Input: part model. Units: mm. Frame: model coordinates. Face numbers are marked on the shaded views. A direction names the side the tool comes from. Coordinates: 2 decimals unless noted, no trailing zeros. Order: outer loops, then holes, each group sorted by start corner. A loop starts at its lowest first (then second) coordinate and runs counter-clockwise, first axis right, second up. Notation, with made-up numbers: (15.25, 6) -> (48.25, 6) arc R8 cw to (48.25, 17) -> close; hole circle Ø8 at (85, 64). An arc over 180 degrees is marked (long way). One line per item, written item: value. Start each with the question number.
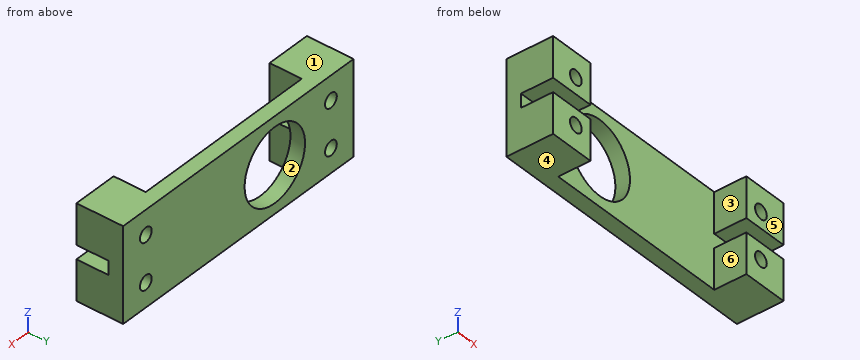
from build123d import *

# Parameters (mm, degrees)
SKETCH2_W           = 61
SKETCH2_H           = 20.5
SKETCH2_R           = 8
SKETCH2_R_2         = 1.55
BOSS_EXTRUDE1_DEPTH = 3.175
SKETCH3_W           = 9.85
SKETCH3_H           = 8.75
SKETCH3_R           = 1.55
BOSS_EXTRUDE2_DEPTH = 7


with BuildPart() as part:
    # Sketch2 → Boss-Extrude1 (new body)
    with BuildSketch(Plane(origin=(0, 0, 0), x_dir=(1, 0, 0), z_dir=(0, 1, 0))):
        Rectangle(SKETCH2_W, SKETCH2_H)
        with Locations((-9.65, 0)):
            Circle(SKETCH2_R, mode=Mode.SUBTRACT)
        with Locations((-24.5, 5)):
            Circle(SKETCH2_R_2, mode=Mode.SUBTRACT)
        with Locations((-24.5, -5)):
            Circle(SKETCH2_R_2, mode=Mode.SUBTRACT)
        with Locations((24.5, 5)):
            Circle(SKETCH2_R_2, mode=Mode.SUBTRACT)
        with Locations((24.5, -5)):
            Circle(SKETCH2_R_2, mode=Mode.SUBTRACT)
    extrude(amount=BOSS_EXTRUDE1_DEPTH)

    # Sketch3 → Boss-Extrude2 (add)
    with BuildSketch(Plane.XZ):
        with Locations((-25.575, 5.875)):
            Rectangle(SKETCH3_W, SKETCH3_H)
        with Locations((-24.5, 5)):
            Circle(SKETCH3_R, mode=Mode.SUBTRACT)
        with Locations((-25.575, -5.875)):
            Rectangle(SKETCH3_W, SKETCH3_H)
        with Locations((-24.5, -5)):
            Circle(SKETCH3_R, mode=Mode.SUBTRACT)
        with Locations((25.575, 5.875)):
            Rectangle(SKETCH3_W, SKETCH3_H)
        with Locations((24.5, 5)):
            Circle(SKETCH3_R, mode=Mode.SUBTRACT)
        with Locations((25.575, -5.875)):
            Rectangle(SKETCH3_W, SKETCH3_H)
        with Locations((24.5, -5)):
            Circle(SKETCH3_R, mode=Mode.SUBTRACT)
    extrude(amount=BOSS_EXTRUDE2_DEPTH)


solid = part.part
1) Section query A-A, the plane y = -5.75. Return the cut outline in (x, z).
2) Section query B-B, the plane x = -24.5. Return the cut outline in (y, z) (3 decimals), plus the area to 3 significant figures.
3) Mould query, pull axis Z, two halves, no side actions, for the marked faces 1, 2, 3 and 4. Classes: +Z half, -Z half, draft (parallel to the pull), parting line (faces both ways), or undercut.
4) Access query for the marked faces 5 and 6. Directions: +Z, -Z, +X, -X, +Y, -Y. A direction counts if a zero-diameter tool reaches every point of the face in a straight line with its end or side. Return the directions, or none.
5) Section query C-C, the plane z = 0. Return the cut outline in (x, y) (3 decimals), plus the area to 3 significant figures.
6) Pin query (flat end, axial travel): pin 1 Ø3 at (x, z) = (17.5, -7.5) entering from -Y. Return the tip coordinate at first contact, or that it passes through.
7) Section query D-D, the plane x = -7.5. Return the cut outline in (y, z) (3 decimals).
8) Ray query, line 1 along X through (y, z) = (-2.5, -5); line 2 along Z through (x, y) = (-24.5, -3.75); line 3 along X through (y, z) = (-2, -8). Return the intervals inside material, ascending. Write a range as from..to.
Entries:
1. outline: (-30.5, -10.25) -> (-20.65, -10.25) -> (-20.65, -1.5) -> (-30.5, -1.5) -> close; (-30.5, 1.5) -> (-20.65, 1.5) -> (-20.65, 10.25) -> (-30.5, 10.25) -> close; (20.65, -10.25) -> (30.5, -10.25) -> (30.5, -1.5) -> (20.65, -1.5) -> close; (20.65, 1.5) -> (30.5, 1.5) -> (30.5, 10.25) -> (20.65, 10.25) -> close; hole circle Ø3.1 at (-24.5, -5); hole circle Ø3.1 at (-24.5, 5); hole circle Ø3.1 at (24.5, -5); hole circle Ø3.1 at (24.5, 5)
2. outline: (-7, -10.25) -> (3.175, -10.25) -> (3.175, -6.55) -> (-7, -6.55) -> close; (-7, -3.45) -> (3.175, -3.45) -> (3.175, 3.45) -> (-7, 3.45) -> (-7, 1.5) -> (0, 1.5) -> (0, -1.5) -> (-7, -1.5) -> close; (-7, 6.55) -> (3.175, 6.55) -> (3.175, 10.25) -> (-7, 10.25) -> close
2. area: 125 mm2
3. face 1: +Z half
3. face 2: undercut
3. face 3: draft
3. face 4: -Z half
4. face 5: +Z, -Z, +X, -X, -Y
4. face 6: +Z, -Z, -Y
5. outline: (-30.5, 0) -> (-17.65, 0) -> (-17.65, 3.175) -> (-30.5, 3.175) -> close; (-1.65, 0) -> (30.5, 0) -> (30.5, 3.175) -> (-1.65, 3.175) -> close
5. area: 143 mm2
6. pin 1: stops at y = 0
7. outline: (0, -10.25) -> (3.175, -10.25) -> (3.175, -7.706) -> (0, -7.706) -> close; (0, 7.706) -> (3.175, 7.706) -> (3.175, 10.25) -> (0, 10.25) -> close
8. line 1: x = -30.5..-26.05, -22.95..-20.65, 20.65..22.95, 26.05..30.5
8. line 2: z = -10.25..-6.55, -3.45..-1.5, 1.5..3.45, 6.55..10.25
8. line 3: x = -30.5..-20.65, 20.65..30.5
